Here's how the part is built. I have some questions about the finished solid (model axes, mm). A direction names the side the tool comes from. Round coordinates to 2 decimals unless told otherwise and drop trailing zeros. Write each loop counter-clockwise with the first axis right and the second up, starting at its lowest first coordinate (ties: lowest second). Pieces come first, ordered by that corner, then holes. Notation, with made-up numbers: (77.25, 64) -> (83.25, 64) arc R4 cw to (83.25, 71) -> close; hole circle Ø3 at (17, -16.5). An arc over 180 degrees is marked (long way). Answer in a Markdown table with one row per item.
from build123d import *

# Parameters (mm, degrees)
SKETCH2_R                       = 23.495
BOSS_EXTRUDE1_DEPTH             = 11.43
SKETCH8_W                       = 3.175
SKETCH8_H                       = 1.905
SKETCH12_R                      = 9.525
BOSS_EXTRUDE2_DEPTH             = 6.35
F_46_0_081_DIAMETER_HOLE1_D     = 2.0574
F_46_0_081_DIAMETER_HOLE1_DEPTH = 17.78


with BuildPart() as part:
    # Sketch2 → Boss-Extrude1 (new body)
    with BuildSketch(Plane(origin=(0, 0, 0), x_dir=(1, 0, 0), z_dir=(0, 1, 0))):
        Circle(SKETCH2_R)
    extrude(amount=BOSS_EXTRUDE1_DEPTH)

    # Sketch8 → Cut-Revolve1 (revolve, cut)
    with BuildSketch(Plane.XY):
        with Locations((19.0373, 10.4775)):
            Rectangle(SKETCH8_W, SKETCH8_H)
    revolve(axis=Axis((0, -0.47625, 0), (0, 1, 0)), mode=Mode.SUBTRACT)

    # Sketch12 → Boss-Extrude2 (add)
    with BuildSketch(Plane.XZ):
        Circle(SKETCH12_R)
    extrude(amount=BOSS_EXTRUDE2_DEPTH)

    # #46 (0.081) Diameter Hole1
    with Locations(Plane(origin=(0, 11.43, 0), x_dir=(1, 0, 0), z_dir=(0, 1, 0))):
        with Locations((-5.715, 0), (-2.568628957, 1.866218176), (0, 0), (-1.766032123, 5.435287991), (4.623532123, 3.359192717), (4.623532123, -3.359192717), (-1.766032123, -5.435287991), (0.981128957, 3.019604439), (3.175, 0), (0.981128957, -3.019604439), (-2.568628957, -1.866218176)):
            Hole(F_46_0_081_DIAMETER_HOLE1_D / 2, depth=F_46_0_081_DIAMETER_HOLE1_DEPTH)


solid = part.part
1) I want a section at C-C, the plane x = -19. List the corners of the cut face in (y, z) for me (3 decimals), and give its area (3 significant figures).
Response:
| item | result |
|---|---|
| outline | (0, -13.821) -> (11.43, -13.821) -> (11.43, -8.024) -> (9.525, -8.024) -> (9.525, 8.024) -> (11.43, 8.024) -> (11.43, 13.821) -> (0, 13.821) -> close |
| area | 285 mm^2 |
2) For pin 1 (1.6 mm diameter, centred on x = 0.98, z = 3.02, fed in from +Y); pin 2 (6 mm diameter, centred on y = 5, z = 5, fed in from -X); pin 3 (3 mm diameter, centred on x = 5.5, z = -18, fed in from -Y); pin 4 (6 mm diameter, centred on x = 8.5, y = 3, fed in from +Z), each with a flat end and sliding along its axis, tell me the tip position at first contact or that it passes through.
Response:
| item | result |
|---|---|
| pin 1 | passes through |
| pin 2 | stops at x = -23.41 |
| pin 3 | stops at y = 0 |
| pin 4 | stops at z = 22.84 |
3) I want a section at A-A, the plane z = 0. List the corners of the cut face in (x, y) for me (3 decimals).
Response:
| item | result |
|---|---|
| outline | (-23.495, 0) -> (-9.525, 0) -> (-9.525, -6.35) -> (-6.744, -6.35) -> (-6.744, 11.43) -> (-17.45, 11.43) -> (-17.45, 9.525) -> (-20.625, 9.525) -> (-20.625, 11.43) -> (-23.495, 11.43) -> close; (-4.686, -6.35) -> (-1.029, -6.35) -> (-1.029, 11.43) -> (-4.686, 11.43) -> close; (1.029, -6.35) -> (2.146, -6.35) -> (2.146, 11.43) -> (1.029, 11.43) -> close; (4.204, -6.35) -> (9.525, -6.35) -> (9.525, 0) -> (23.495, 0) -> (23.495, 11.43) -> (20.625, 11.43) -> (20.625, 9.525) -> (17.45, 9.525) -> (17.45, 11.43) -> (4.204, 11.43) -> close |
4) I want a section at D-D, the plane z = -11. List the corners of the cut face in (x, y) for me (3 decimals), and give its area (3 significant figures).
Response:
| item | result |
|---|---|
| outline | (-20.761, 0) -> (20.761, 0) -> (20.761, 11.43) -> (17.447, 11.43) -> (17.447, 9.525) -> (13.546, 9.525) -> (13.546, 11.43) -> (-13.546, 11.43) -> (-13.546, 9.525) -> (-17.447, 9.525) -> (-17.447, 11.43) -> (-20.761, 11.43) -> close |
| area | 460 mm^2 |
5) We'd pull the mould along X, two halves only. Please class faces 3 (the face through (0, 0, 10)), 4 (the face through (-1.75, 2.42, -1.24)), 5 (the face through (1.12, 2.42, -4.04)), 6 (the face through (-7.559, -3.131, -5.796)): +X half, -X half, draft (parallel to the pull), parting line (faces both ways), or undercut.
Response:
| item | result |
|---|---|
| face 3 | draft |
| face 4 | undercut |
| face 5 | undercut |
| face 6 | parting line |
6) I want a section at B-B, the plane y = 6.25. Count the separate pieces of the cut face and the enclosed holes in it, and give its area (3 significant figures).
Response:
| item | result |
|---|---|
| separate pieces | 1 |
| enclosed holes | 11 |
| area | 1,700 mm^2 |
7) I need wall thicknesses on line 1 (Z direction, x = 0.5, y = 1.5); line 2 (X direction, y = 0.25, z = 3); line 3 (Z direction, x = -2, y = -2.25). Which ranges of each line are inside material? Lowest first, please. Write a range as [from, to].
Response:
| item | result |
|---|---|
| line 1 | z = [-23.49, -3.93], [-2.11, -0.9], [0.9, 2.11], [3.93, 23.49] |
| line 2 | x = [-23.3, -0.05], [2.01, 3.66], [5.59, 23.3] |
| line 3 | z = [-9.31, -6.44], [-4.43, -2.72], [-1.01, 1.01], [2.72, 4.43], [6.44, 9.31] |
8) Which directions (+Z, -Z, +X, -X, +Y, -Y) give clear straight access to the entire face, cutting with the end or side of a thin tool? Please do faces 1 (the face through (-1.54, 2.42, -4.43)), 2 (the face through (17, 9.525, -5)).
Response:
| item | result |
|---|---|
| face 1 | +Y, -Y |
| face 2 | +Y |
